The listing builds one solid part. Answer for the finished solid, in the listing's coordinates (mm). A direction names the side the tool comes from. Round coordinates to 2 decimals unless told otherwise and drop trailing zeros. Write each loop counter-clockwise with the first axis right and the second up, starting at its lowest first coordinate (ties: lowest second). Pieces come first, ordered by that corner, then holes. Notation, with made-up numbers: M 6,3.25 L 25,3.25 A16 ccw 25,19.25 Z; hole C 75.5,-19 d3. An arc over 180 degrees is marked long. One line per item, written item: value. Start each with the question number.
(1) Section C-C (y = 4) is taken. Determine the outline of the cut face in (x, z), plus the area to 3 significant figures.
(2) Section D-D (z = -15) is taken. Determine the outline of the cut face in (x, y), plus the area to 3 significant figures.
(3) For faces 5 (the flat face through (-3, 34.29, 2)), 6 (the cylindrical face through (17.37, 1.25, 3.26)), 7 (the flat face through (4.7, 2.54, -9.2)), 8 (the cylindrical face through (-1.93, 1.29, -2.52)), 9 (the cylindrical face through (-1.396, 27.351, -5.145)), determine the directions among +Z, -Z, +X, -X, +Y, -Y from which every point of the face is accessible in a straight line to the end or side of a thin tool.
(4) Consider probe 1 along X at (y, z) = (1, 0) (3 decimals); probe 2 along Y at (x, z) = (-6, 0); probe 3 along Y at (x, z) = (-11.5, 3.5). Determine where each line is inside the solid, lowest interval first.
(5) For a pull along X with two mould halves and no side action, classify faces 1 (the cylindrical face through (-6.888, 1.252, -16.628)), 2 (the cylindrical face through (-5.145, 22.351, 1.396)), 3 (the flat face through (0, 2.54, 0)), 4 (the cylindrical face through (-19.524, 1.252, -4.336)) as released by +X, released by -X, zero draft, split by the parting line, or undercut.
(6) Section A-A (z = 0) is taken. Determine the outline of the cut face in (x, y) (3 decimals), plus the area to 3 significant figures.
(7) Section B-B (x = 17) is taken. Determine the outline of the cut face in (y, z).
(8) Given P1, Ø10, axis at x = 9.5, z = 12, coming from the -Y side; P2, Ø4, axis at x = 3.5, y = 27.5, coming from the +Z side; P3, Ø5, axis at x = -10.04, z = 13.09, coming from the +Y side; P4, Ø1.5, axis at y = 14, z = 6, coming from the +X side, each flat-ended and moving along its own axis, determine where each tip first touches the part or whether it passes through.
```python
from build123d import *

# Parameters (mm, degrees)
SKETCH1_R           = 20
BOSS_EXTRUDE1_DEPTH = 2.54
SKETCH2_R           = 7.499999986
BOSS_EXTRUDE2_DEPTH = 31.75
SKETCH6_R           = 1.5
CUT_EXTRUDE2_DEPTH  = 45.450017998
SKETCH7_R           = 3.175
CUT_EXTRUDE3_DEPTH  = 45.450017998
SKETCH8_R           = 1.397
CUT_EXTRUDE4_DEPTH  = 45.450017998
SKETCH9_R           = 1.397
CUT_EXTRUDE5_DEPTH  = 45.450018075
SKETCH10_R          = 10.16
BOSS_EXTRUDE3_DEPTH = 5.08


with BuildPart() as part:
    # Sketch1 → Boss-Extrude1 (new body)
    with BuildSketch(Plane(origin=(0, 0, 0), x_dir=(1, 0, 0), z_dir=(0, 1, 0))):
        with Locations(Location((0, 0, 0), (0, 0, 270))):
            Circle(SKETCH1_R)
    extrude(amount=BOSS_EXTRUDE1_DEPTH)

    # Sketch2 → Boss-Extrude2 (add)
    with BuildSketch(Plane(origin=(0, 2.54, 0), x_dir=(1, 0, 0), z_dir=(0, 1, 0))):
        with Locations(Location((0, 0, 0), (0, 0, 270))):
            Circle(SKETCH2_R)
    extrude(amount=BOSS_EXTRUDE2_DEPTH)

    # Sketch6 → Cut-Extrude2 (cut, through all)
    with BuildSketch(Plane(origin=(0, 0, 0), x_dir=(-1, 0, 0), z_dir=(0, -1, 0))):
        with Locations(Location((6.313805851, 15.242875716, 0), (0, 0, 90))):
            Circle(SKETCH6_R)
        with Locations(Location((10.043814672, -13.08935412, 0), (0, 0, 90))):
            Circle(SKETCH6_R)
        with Locations(Location((-16.357620523, -2.153521596, 0), (0, 0, 90))):
            Circle(SKETCH6_R)
    extrude(amount=-CUT_EXTRUDE2_DEPTH, mode=Mode.SUBTRACT)

    # Sketch7 → Cut-Extrude3 (cut, through all)
    with BuildSketch(Plane(origin=(0, 34.29, 0), x_dir=(1, 0, 0), z_dir=(0, 1, 0))):
        with Locations(Location((0, 0, 0), (0, 0, 270))):
            Circle(SKETCH7_R)
    extrude(amount=-CUT_EXTRUDE3_DEPTH, mode=Mode.SUBTRACT)

    # Sketch8 → Cut-Extrude4 (cut, through all)
    with BuildSketch(Plane(origin=(0, 0, 0), x_dir=(0, 0, -1), z_dir=(1, 0, 0))):
        with Locations((0, 22.29)):
            Circle(SKETCH8_R)
    extrude(amount=-CUT_EXTRUDE4_DEPTH, mode=Mode.SUBTRACT)

    # Sketch9 → Cut-Extrude5 (cut, through all)
    with BuildSketch(Plane.XY):
        with Locations((0, 27.29)):
            Circle(SKETCH9_R)
    extrude(amount=-CUT_EXTRUDE5_DEPTH, mode=Mode.SUBTRACT)

    # Sketch10 → Boss-Extrude3 (add)
    with BuildSketch(Plane(origin=(0, 2.54, 0), x_dir=(1, 0, 0), z_dir=(0, 1, 0))):
        with Locations(Location((0, 0, 0), (0, 0, 270))):
            Circle(SKETCH10_R)
    extrude(amount=BOSS_EXTRUDE3_DEPTH)


solid = part.part
```
Recorded:
1. outline: C 0,0 d20.32
1. area: 324 mm2
2. outline: M -13.23,0 L -7.79,0 L -7.79,2.54 L -13.23,2.54 Z; M -4.83,0 L 13.23,0 L 13.23,2.54 L -4.83,2.54 Z
2. area: 59.7 mm2
3. face 5: +Z, -Z, +X, -X, +Y
3. face 6: +Y, -Y
3. face 7: +Y
3. face 8: -Y
3. face 9: -Z
4. probe 1: x = -20 to -3.175, 3.175 to 20
4. probe 2: y = 0 to 20.89, 23.69 to 34.29
4. probe 3: y = 0 to 2.54
5. face 1: undercut
5. face 2: zero draft
5. face 3: undercut
5. face 4: split by the parting line
6. outline: M -20,0 L -3.175,0 L -3.175,2.54 L 3.175,2.54 L 3.175,0 L 20,0 L 20,2.54 L 10.16,2.54 L 10.16,7.62 L 7.5,7.62 L 7.5,34.29 L 3.175,34.29 L 3.175,7.62 L -3.175,7.62 L -3.175,20.893 L -7.5,20.893 L -7.5,7.62 L -10.16,7.62 L -10.16,2.54 L -20,2.54 Z; M -7.5,23.687 L -3.175,23.687 L -3.175,34.29 L -7.5,34.29 Z
6. area: 407 mm2
7. outline: M 0,-10.54 L 2.54,-10.54 L 2.54,0.8 L 0,0.8 Z; M 0,3.51 L 2.54,3.51 L 2.54,10.54 L 0,10.54 Z
8. P1: stops at y = 0
8. P2: stops at z = 7.35
8. P3: stops at y = 2.54
8. P4: stops at x = 5.36
